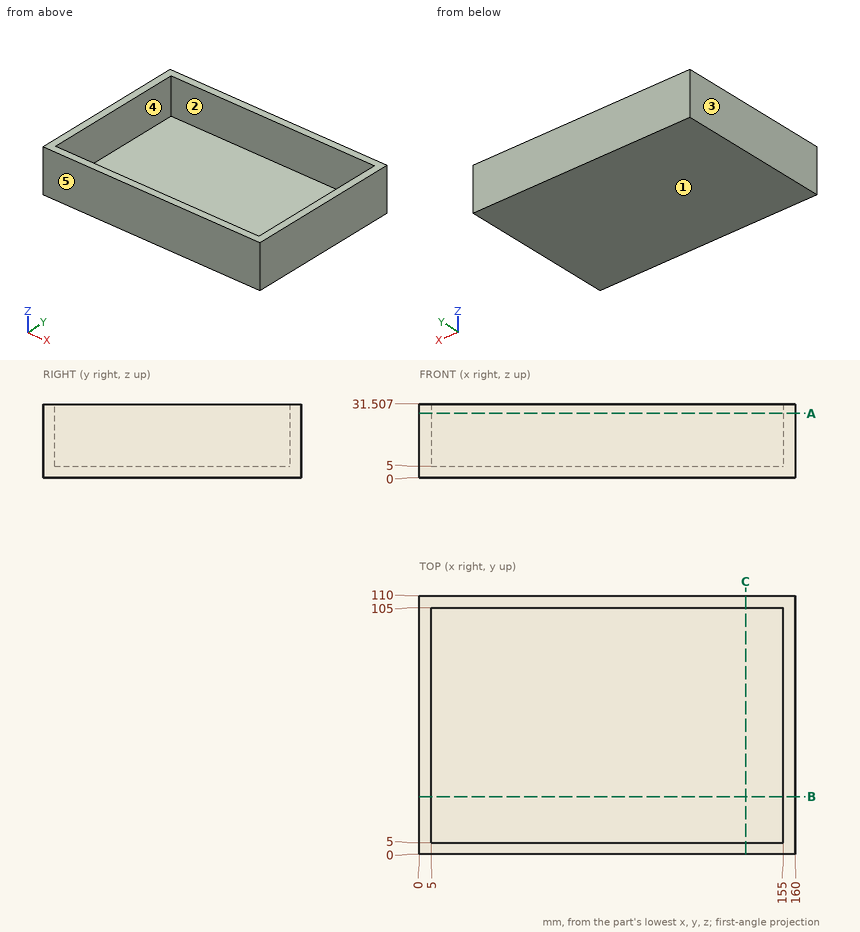
Here's the drawing with two shaded views (mm, measured from the low corner). I have some questions. A direction names the side the tool comes from. Give positions to 0.01 mm unless a question says otherwise; leave off trailing zeros. Order: outer loops, then holes, each group sorted by start corner. A loop starts at its lowest first (then second) coordinate and runs counter-clockwise, first axis right, second up. Notation, with made-up numbers: (51, 44) -> (64, 44) arc R33 ccw to (64, 80) -> close; hole circle Ø5 at (23.25, -13.5). An arc over 180 degrees is marked (long way). One line per item, written item: value. Start each with the question number.
1. Will this pin go through, and if not, where does the flat tip stop? pin 1 Ø5 at (x, z) = (111.5, 26.5) entering from -Y.
2. For the marked faces 4 and 5, which set-ups out of +Z, -Z, +X, -X, +Y, -Y let a thin tool reach every point of the face, with its end or its side?
3. We'd pull the mould along X, two halves only. Please class the marked faces 1, 2 and 3: released by +X, released by -X, zero draft, split by the parting line, or undercut.
4. Imagine slicing it at C-C, the plane x = 139. List the corners of the cut face in (y, z) for me, plus the area to 3 significant figures.
5. Imagine slicing it at A-A, the plane z = 27.5. List the corners of the cut face in (x, y) for me.
6. Imagine slicing it at B-B, the plane y = 24.5. List the corners of the cut face in (x, z) for me.
7. I need wall thicknesses on probe 1 along X at (y, z) = (17.5, 23); probe 2 along Y at (x, z) = (107, 5.5); probe 3 along Z at (x, y) = (40, 42). Which ranges of each line are inside material? Lowest first, please. Write a range as from..to.
Values follow:
1. pin 1: stops at y = 0
2. face 4: +Z
2. face 5: +Z, -Z, +X, -X, -Y
3. face 1: zero draft
3. face 2: undercut
3. face 3: released by -X
4. outline: (0, 0) -> (110, 0) -> (110, 31.51) -> (105, 31.51) -> (105, 5) -> (5, 5) -> (5, 31.51) -> (0, 31.51) -> close
4. area: 815 mm2
5. outline: (0, 0) -> (160, 0) -> (160, 110) -> (0, 110) -> close; hole (5, 5) -> (155, 5) -> (155, 105) -> (5, 105) -> close
6. outline: (0, 0) -> (160, 0) -> (160, 31.51) -> (155, 31.51) -> (155, 5) -> (5, 5) -> (5, 31.51) -> (0, 31.51) -> close
7. probe 1: x = 0..5, 155..160
7. probe 2: y = 0..5, 105..110
7. probe 3: z = 0..5
